```python
from build123d import *

# Parameters (mm, degrees)
F0_W     = 9.4565711915
F0_H     = 13.6675285175
F1_DEPTH = 15.3
F2_W     = 109.1410517693
F2_H     = 22.5323475897
F3_DEPTH = 77
F4_R     = 2.5676865252
F5_DEPTH = 65.4
F6_R     = 1.5468397632
F7_DEPTH = 54.6
F8_R     = 2.6556349186
F9_R     = 1
F10_R    = 0.0237853743


with BuildPart() as f1:
    # F0 (on Top) → F1 (new body)
    with BuildSketch(Plane.XY):
        Polygon((-40.6965725124, 44.3279668689), (-43.8004508615, 44.3550609052), (-43.8004508615, 25.7457569242), (-53.257022053, 25.7457569242), (-53.257022053, 44.6070879698), (-57.4438385665, 44.6070879698), (-57.4438385665, 21.5618759394), (-67.321151495, 31.8517945707), (-67.321151495, 44.6070879698), (-72.1341744065, 44.6070879698), (-72.1341744065, 31.8517945707), (-57.4438385665, 15.2993714437), (-57.4438385665, -7.5885597616), (-70.2834129333, -20.1490093023), (-70.2834129333, -50.7155247033), (-57.4438385665, -50.7155247033), (-57.4438385665, -38.6135876179), (-43.8004508615, -38.6135876179), (-43.8004508615, -50.7155247033), (-36.5097559988, -50.7155247033), (-36.5097559988, -35.2215506136), (-40.6965725124, -28.8017634302), align=None)
        Polygon((-43.8004508615, -10.5956946412), (-43.8004508615, -35.2215506136), (-57.4438385665, -35.2215506136), (-57.4438385665, -14.0083450824), (-55.5479216548, -10.5956946412), align=None, mode=Mode.SUBTRACT)
        Polygon((-49.6741862581, -7.5885597616), (-53.257022053, -7.5885597616), (-53.257022053, 4.3360902928), (-49.6741862581, 4.3360902928), (-43.8004508615, 4.3360902928), (-43.8004508615, -7.5885597616), align=None, mode=Mode.SUBTRACT)
        with Locations((-48.5287364572, 14.5968659781)):
            Rectangle(F0_W, F0_H, mode=Mode.SUBTRACT)
    extrude(amount=F1_DEPTH)

    # F2 (on face) → F3 (cut)
    with BuildSketch(Plane(origin=(-72.1341744065, 0, 0), x_dir=(0, -1, 0), z_dir=(-1, 0, 0))):
        with Locations((3.7736594677, 6.6085606813)):
            Rectangle(F2_W, F2_H)
        with BuildLine():
            ThreePointArc((39.6816573, 14.1380049634), (44.9345471885, 12.1822751735), (47.1420204778, 7.0301112719))
            ThreePointArc((47.1420204778, 7.0301112719), (44.6510850499, 1.622031227), (38.9221144813, 0))
            Line((38.9221144813, 0), (-31.8517945707, 0))
            Line((-31.8517945707, 0), (-37.1405081916, 0))
            ThreePointArc((-37.1405081916, 0), (-38.2294412702, -0.1143932508), (-39.3183743488, 0))
            Line((-39.3183743488, 0), (-44.6070879698, 0))
            Line((-44.6070879698, 0), (-44.6070879698, 15.3))
            Line((-44.6070879698, 15.3), (-31.8517945707, 15.3))
            Line((-31.8517945707, 15.3), (-31.8517945707, 10.6745666141))
            Line((-31.8517945707, 10.6745666141), (39.6816573, 14.1380049634))
        make_face(mode=Mode.SUBTRACT)
    extrude(amount=-F3_DEPTH, mode=Mode.SUBTRACT)

    # F4 (on face) → F5 (cut)
    with BuildSketch(Plane(origin=(-72.1341744065, 0, 0), x_dir=(0, -1, 0), z_dir=(-1, 0, 0))):
        with Locations((40.1412695646, 6.1273775063)):
            Circle(F4_R)
    extrude(amount=-F5_DEPTH, mode=Mode.SUBTRACT)

    # F6 (on face) → F7 (cut)
    with BuildSketch(Plane(origin=(-72.1341744065, 0, 0), x_dir=(0, -1, 0), z_dir=(-1, 0, 0))):
        with Locations((-36.5287549794, 6.0891942121)):
            Circle(F6_R)
    extrude(amount=-F7_DEPTH, mode=Mode.SUBTRACT)

    # F8
    f8_edges = [f1.edges().sort_by_distance(p)[0] for p in [
        (-56.49588, -12.30202, 0),
        (-55.547922, -10.595695, 6.364874),
        (-56.49588, -12.30202, 12.812364),
        (-57.443839, -14.008345, 6.44749),
        (-49.674186, -10.595695, 0),
        (-57.443839, -24.614948, 0),
        (-49.674186, -10.595695, 12.729749),
        (-57.443839, -24.614948, 13.408519),
    ]]
    fillet(f8_edges, radius=F8_R)

    # F9
    f9_edges = [f1.edges().sort_by_distance(p)[0] for p in [
        (-63.863626, -13.868785, 0),
        (-70.283413, -20.149009, 6.596146),
        (-63.863626, -13.868785, 12.888222),
        (-57.443839, -7.58856, 6.292076),
        (-57.443839, 3.855406, 0),
        (-57.443839, 3.855406, 12.030069),
    ]]
    fillet(f9_edges, radius=F9_R)

    # F10
    f10_edges = [f1.edges().sort_by_distance(p)[0] for p in [
        (-40.696573, 44.327967, 7.65),
        (-43.800451, 44.355061, 7.65),
        (-42.248512, 44.341514, 0),
        (-42.248512, 44.341514, 15.3),
    ]]
    fillet(f10_edges, radius=F10_R)


solid = f1.part
```
Input: part model. Units: mm. Frame: model coordinates. A direction names the side the tool comes from. Coordinates: 2 decimals unless noted, no trailing zeros. Loops run counter-clockwise (first coordinate to the right, second up) from the corner with the lowest first, then second, coordinate; pieces in that order, holes last. Notation, with made-up numbers: M 67.25,79.25 L 123.25,79.25 A19 ccw 123.25,112.25 Z; hole C 4.25,69.25 d11. An arc over 180 degrees is marked long. Answer in a Markdown table with one row per item.
1. Section B-B, the plane y = 17. Output: boundary loops of the cut face in (x, z).
Response:
| item | result |
|---|---|
| outline | M -58.95,0 L -53.26,0 L -53.26,11.39 L -58.95,11.39 Z; M -43.8,0 L -40.7,0 L -40.7,11.39 L -43.8,11.39 Z |
2. Section A-A, the plane x = -52. Output: boundary loops of the cut face in (y, z).
Response:
| item | result |
|---|---|
| outline | M -38.61,0 L -35.22,0 L -35.22,13.92 L -38.61,14.09 L -38.61,8.19 A2.57 cw -38.61,4.06 Z; M -10.6,2.66 A2.66 ccw -7.94,0 L -7.59,0 L -7.59,12.58 L -7.81,12.59 A2.66 ccw -10.6,9.94 Z; M 4.34,0 L 7.76,0 L 7.76,11.84 L 4.34,12.01 Z; M 21.43,0 L 25.75,0 L 25.75,10.97 L 21.43,11.18 Z |
3. First-contact query: pin 1 (1.5 mm diameter, centred on x = -53.5, y = 10.5, fed in from +Z); pin 2 (2 mm diameter, centred on x = -54.5, z = 11.5, fed in from -Y); pin 3 (1 mm diameter, centred on x = -64.5, z = 8, fed in from +Y). Flat tips, straight axial feed; report the tip coordinate or a pass-through.
Response:
| item | result |
|---|---|
| pin 1 | stops at z = 11.74 |
| pin 2 | stops at y = -38.61 |
| pin 3 | stops at y = 29.43 |
4. Section C-C, the plane x = -66. Count the separate pieces of the cut face and the enclosed holes in it, then the cut area to 3 significant figures.
Response:
| item | result |
|---|---|
| separate pieces | 2 |
| enclosed holes | 1 |
| area | 445 mm2 |
5. Section D-D, the plane x = -39.5. Output: boundary loops of the cut face in (y, z).
Response:
| item | result |
|---|---|
| outline | M -41.13,0 L -30.64,0 L -30.64,13.7 L -39.68,14.14 A7.12 ccw Z; hole C -40.14,6.13 d5.14 |
6. Reachability of faces 5 (the flat face through (-43.8, -43, 7)), 6 (the cylindrical face through (-48.82, -9.8, 0.76)), 7 (the cylindrical face through (-57.39, -12.22, 12.03)) from +Z, -Z, +X, -X, +Y, -Y: full face, straight path, thin tool, end or side. Return the list, or none.
Response:
| item | result |
|---|---|
| face 5 | +Z, -Z, -Y |
| face 6 | -Z |
| face 7 | +Z |
7. Draft query along X for faces 1 (the cylindrical face through (-48.964, -9.75, 11.886)), 2 (the flat face through (-62.31, 26.63, 5.51)), 3 (the flat face through (-55, 44.607, 8)), 4 (the flat face through (-40.697, 7, 6)). Return one class per face: pulls with the +X half, pulls with the -X half, needs draft (parallel to the pull), parting line crosses it, or undercut.
Response:
| item | result |
|---|---|
| face 1 | undercut |
| face 2 | undercut |
| face 3 | needs draft |
| face 4 | pulls with the +X half |
8. Material intervals for line 1 (X direction, y = 32.5, z = 14); line 2 (Y direction, x = -51, z = 9.5); line 3 (X direction, y = 4, z = 2.25), sorted ascending.
Response:
| item | result |
|---|---|
| line 1 | x = -72.13 to -67.32, -57.44 to -53.26, -43.8 to -40.7 |
| line 2 | y = -38.61 to -35.22, -10.6 to -7.59, 4.34 to 7.76, 21.43 to 25.75 |
| line 3 | x = -57.44 to -53.26, -43.8 to -40.7 |
